Input: part model. Units: mm. Frame: model coordinates. A direction names the side the tool comes from. Give positions to 0.01 mm unless a question says otherwise; leave off trailing zeros. Loops run counter-clockwise (first coordinate to the right, second up) from the corner with the lowest first, then second, coordinate; pieces in that order, holes last. Notation, with made-up numbers: (-16.5, 5) -> (22.5, 5) arc R18 cw to (22.5, 11) -> close; hole circle Ø5 at (35.5, -5.5). An arc over 180 degrees is marked (long way). Use CSV: the item, a comma, the result in double quotes.
```python
from build123d import *

# Parameters (mm, degrees)
F0_R          = 10.5
F1_DEPTH      = 110
F2_W          = 9
F2_H          = 9
F3_DEPTH      = 5
F6_DEPTH      = 10.5
F6_DEPTH_BACK = 10.5
F7_R          = 7.5
F8_DEPTH      = 5
F8_DEPTH_BACK = 25


with BuildPart() as f1:
    # F0 (on Top) → F1 (new body)
    with BuildSketch(Plane.XY):
        Circle(F0_R)
    extrude(amount=F1_DEPTH)

    # F2 (on Top) → F3 (join)
    with BuildSketch(Plane.XY):
        Rectangle(F2_W, F2_H)
    extrude(amount=-F3_DEPTH)

    # F4 (on Right) → F6 (join, two sides)
    with BuildSketch(Plane.YZ) as f6_sk:
        Polygon((-12.8786796564, 0), (0, 0), (0, 17.1421356237), (-4.0398448916, 17.1421356237), (-7.5753787975, 17.1421356237), (-12.8786796564, 11.8388347648), (-18.1819805153, 6.5355339059), (-21.1819805153, 6.5355339059), (-21.1819805153, 0), align=None)
    extrude(amount=F6_DEPTH)
    extrude(f6_sk.sketch, amount=-F6_DEPTH_BACK)

    # F7 (on face) → F8 (cut, two sides)
    with BuildSketch(Plane(origin=(0, -12.3587572106, 12.3587572106), x_dir=(1, 0, 0), z_dir=(0, -0.7071067812, 0.7071067812))) as f8_sk:
        with Locations((0, -0.7352813742)):
            Circle(F7_R)
    extrude(amount=-F8_DEPTH, mode=Mode.SUBTRACT)
    extrude(f8_sk.sketch, amount=F8_DEPTH_BACK, mode=Mode.SUBTRACT)


solid = f1.part
```
1) Contact query for flat-ended pins moving along their axis: pin 1 (4 mm diameter, centred on x = -0.5, z = -3, fed in from +Y); pin 2 (1.5 mm diameter, centred on x = 3.5, z = 12, fed in from -Y); pin 3 (1.5 mm diameter, centred on x = 1.5, y = -6.5, fed in from -Z). Output: stop coordinate, or through.
From the geometry:
pin 1,"stops at y = 4.5"
pin 2,"stops at y = -6.4"
pin 3,"stops at z = 0"
2) Ray query, line 1 (Z direction, x = -4, y = 5); line 2 (Z direction, x = -5.5, y = -6); line 3 (Z direction, x = -2.5, y = -8). Return the intervals inside material, ascending.
From the geometry:
line 1,"z = 0 to 110"
line 2,"z = 0 to 11.65, 12.17 to 110"
line 3,"z = 0 to 9.65, 16.96 to 110"
3) Section query B-B (x = 8.75). Return loops of the section in (y, z).
From the geometry:
outline,"(-21.18, 0) -> (5.8, 0) -> (5.8, 110) -> (-5.8, 110) -> (-5.8, 17.14) -> (-7.58, 17.14) -> (-18.18, 6.54) -> (-21.18, 6.54) -> close"
4) Reachability of faces 4 (the flat face through (0, -20, 6.536)), 5 (the flat face through (4.5, 0, -2)), 6 (the cylindrical face through (-1.37, 10.41, 54.23)), 7 (the flat face through (0, -4.5, -2)) from +Z, -Z, +X, -X, +Y, -Y: full face, straight path, thin tool, end or side. Return the list, or none.
From the geometry:
face 4,"+Z, +X, -X, -Y"
face 5,"-Z, +X, +Y, -Y"
face 6,"+Z"
face 7,"-Z, +X, -X, -Y"
5) Mould query, pull axis Z, two halves, no side actions, for faces 1 (the flat face through (9, -6, 17.142)), 2 (the flat face through (-0.105, -9.269, 8.378)), 3 (the flat face through (0, 4.5, -2)). Classes: pulls with the +Z half, pulls with the -Z half, needs draft (parallel to the pull), parting line crosses it, or undercut.
From the geometry:
face 1,"pulls with the +Z half"
face 2,"undercut"
face 3,"needs draft"
6) Section query A-A (y = -3). Return loops of the section in (x, z).
From the geometry:
outline,"(-10.5, 0) -> (-4.5, 0) -> (-4.5, -5) -> (4.5, -5) -> (4.5, 0) -> (10.5, 0) -> (10.5, 17.14) -> (10.06, 17.14) -> (10.06, 110) -> (-10.06, 110) -> (-10.06, 17.14) -> (-10.5, 17.14) -> close"
7) Section query C-C (z = 80). Return loops of the section in (x, y), then the cut area to 3 significant figures.
From the geometry:
outline,"circle Ø21 at (0, 0)"
area,"346 mm^2"
